Model file for the job. Use its own axes, mm. A direction names the side the tool comes from. Give positions to 0.01 mm unless a question says otherwise; leave off trailing zeros. Loops run counter-clockwise (first coordinate to the right, second up) from the corner with the lowest first, then second, coordinate; pieces in that order, holes last. Notation, with made-up numbers: (-11, 43) - (40, 43) arc R13 ccw to (40, 52) - close; hole circle Ø2 at (-19, 84.25). An arc over 180 degrees is marked (long way). Use a Markdown table: item, result.
from build123d import *

# Parameters (mm, degrees)
F0_W     = 190.5
F0_H     = 101.6
F1_DEPTH = 177.8
F3_DEPTH = 101.601


with BuildPart() as f1:
    # F0 (on Front) → F1 (new body)
    with BuildSketch(Plane.XZ):
        Rectangle(F0_W, F0_H)
    extrude(amount=F1_DEPTH)

    # F2 (on face) → F3 (cut, through all)
    with BuildSketch(Plane(origin=(0, 0, -50.8), x_dir=(1, 0, 0), z_dir=(0, 0, -1))):
        Polygon((-95.25, 177.8), (-95.25, 50.8), (-82.55, 50.8), (-9.226516, 177.8), align=None)
    extrude(amount=-F3_DEPTH, mode=Mode.SUBTRACT)


solid = f1.part
(1) Pin check, flat tips, straight feed: P1, Ø4, axis at x = -92, z = -18.5, coming from the -Y side; P2, Ø6, axis at y = -137.5, z = -11.5, coming from the -X side. Stop position of each tip, or through.
Computed:
| item | result |
|---|---|
| P1 | y = -50.8 |
| P2 | x = -34.23 |
(2) Mould opens along X. For faces 3 (the flat face through (-95.25, -25, -1)), 4 (the flat face through (95.25, -88, -1)), 5 (the flat face through (42, -177.8, 1)) say: pulls with the +X half, pulls with the -X half, needs draft (parallel to the pull), parting line crosses it, or undercut.
Computed:
| item | result |
|---|---|
| face 3 | pulls with the -X half |
| face 4 | pulls with the +X half |
| face 5 | needs draft |
(3) Slice it at A-A, the plane z = -27.5. Write the cut outline in (x, y), plus the area to 3 significant figures.
Computed:
| item | result |
|---|---|
| outline | (-95.25, -50.8) - (-82.55, -50.8) - (-9.23, -177.8) - (95.25, -177.8) - (95.25, 0) - (-95.25, 0) - close |
| area | 27,600 mm² |
(4) Slice it at C-C, the plane x = -49. Write the cut outline in (y, z).
Computed:
| item | result |
|---|---|
| outline | (-108.91, -50.8) - (0, -50.8) - (0, 50.8) - (-108.91, 50.8) - close |
(5) Slice it at B-B, the plane y = -96.5. Write the cut outline in (x, z).
Computed:
| item | result |
|---|---|
| outline | (-56.17, -50.8) - (95.25, -50.8) - (95.25, 50.8) - (-56.17, 50.8) - close |
(6) Drill centre lines: probe 1 along X at (y, z) = (-116.5, -17); probe 2 along Y at (x, z) = (-82.5, -33); probe 3 along X at (y, z) = (-126, 41). Where is each one in solid material? Low to high. Write a range as [from, to].
Computed:
| item | result |
|---|---|
| probe 1 | [-44.62, 95.25] |
| probe 2 | [-50.89, 0] |
| probe 3 | [-39.13, 95.25] |
(7) 3-axis set-ups, long thin cutter, end or side, ignore diameter. For faces 1 (the flat face through (-1, 0, 1)), 2 (the flat face through (-89, -50.8, -1)): which of +Z, -Z, +X, -X, +Y, -Y reach the whole face in a straight line?
Computed:
| item | result |
|---|---|
| face 1 | +Z, -Z, +X, -X, +Y |
| face 2 | +Z, -Z, -X, -Y |
